Read the model definition and answer for the solid it produces. Units are mm, in the model's axes. A direction names the side the tool comes from. Round coordinates to 2 decimals unless told otherwise and drop trailing zeros. Write each loop counter-clockwise with the first axis right and the second up, starting at its lowest first coordinate (ties: lowest second). Pieces come first, ordered by that corner, then holes. Notation, with made-up numbers: M 27,16 L 42,16 A16 ccw 42,40 Z; hole C 60,87.5 d8. An arc over 180 degrees is marked long. Use one line per item in the form item = value. Start each with the question number.
```python
from build123d import *

# Parameters (mm, degrees)
SKETCH_1_R          = 1.8000000000000025
SKETCH_1_R_2        = 1.8000000000000043
SKETCH_1_R_3        = 1.8000000000000005
SKETCH_1_R_4        = 1.8000000000000007
EXTRUDE_1_DEPTH     = 42
SKETCH_2_R          = 6.000000000000001
CUT_EXTRUDE_1_DEPTH = 58.404268133998535
SKETCH_3_R          = 6.000000000000002
CUT_EXTRUDE_2_DEPTH = 58.404268133998535
SKETCH_5_W          = 12
SKETCH_5_H          = 15.000000000000005
SKETCH_5_H_2        = 15.000000000000002
CUT_EXTRUDE_3_DEPTH = 58.404268133998535
EXTRUDE_2_DEPTH     = 2.1
EXTRUDE_3_DEPTH     = 1
EXTRUDE_START       = 2.1
EXTRUDE_4_DEPTH     = 2.1
EXTRUDE_START_2     = 1
EXTRUDE_5_DEPTH     = 1
SKETCH_10_R         = 1.5000000000000018
CUT_EXTRUDE_4_DEPTH = 3


with BuildPart() as part:
    # 草图1 → 凸台-拉伸1 (new body)
    with BuildSketch(Plane(origin=(0, 0, 0), x_dir=(-1, 0, 0), z_dir=(0, 0, 1))):
        with BuildLine():
            Line((-17.499999999999996, 15), (-17.499999999999996, -15.000000000000007))
            ThreePointArc((-17.499999999999996, -15.000000000000007), (-16.767766952966365, -16.767766952966372), (-15, -17.500000000000007))
            Line((-15, -17.500000000000007), (15.000000000000004, -17.500000000000007))
            ThreePointArc((15.000000000000004, -17.500000000000007), (16.76776695296637, -16.767766952966376), (17.5, -15.00000000000001))
            Line((17.5, -15.00000000000001), (17.5, 14.999999999999996))
            ThreePointArc((17.5, 14.999999999999996), (16.76776695296637, 16.76776695296636), (15.000000000000004, 17.499999999999996))
            Line((15.000000000000004, 17.499999999999996), (-15, 17.499999999999996))
            ThreePointArc((-15, 17.499999999999996), (-16.767766952966365, 16.767766952966365), (-17.499999999999996, 15))
        make_face()
        with Locations((-15.000000000000004, -15.00000000000001)):
            Circle(SKETCH_1_R, mode=Mode.SUBTRACT)
        with Locations((15.000000000000004, -15.00000000000001)):
            Circle(SKETCH_1_R_2, mode=Mode.SUBTRACT)
        with Locations((15.000000000000004, 14.999999999999996)):
            Circle(SKETCH_1_R_3, mode=Mode.SUBTRACT)
        with Locations((-15, 15)):
            Circle(SKETCH_1_R_4, mode=Mode.SUBTRACT)
        with BuildLine():
            Line((15.604722413530899, -11.417049414734192), (15.604722413530899, 11.41704941481964))
            ThreePointArc((15.604722413530899, 11.41704941481964), (15.349600753639777, 12.084241863325458), (14.714404940145743, 12.41098197902667))
            ThreePointArc((14.714404940145743, 12.41098197902667), (13.158183898644735, 13.15818233801838), (12.410982220986185, 14.714402746377065))
            ThreePointArc((12.410982220986185, 14.714402746377065), (12.084242685294747, 15.349600017363324), (11.417049414775391, 15.604722413530212))
            Line((11.417049414775391, 15.604722413530212), (-11.417049414778536, 15.604722413530212))
            ThreePointArc((-11.417049414778536, 15.604722413530212), (-12.084241863278942, 15.349600753643644), (-12.410981978984013, 14.714404940159108))
            ThreePointArc((-12.410981978984013, 14.714404940159108), (-13.158182337972896, 13.158183898648431), (-14.714402746337697, 12.41098222098531))
            ThreePointArc((-14.714402746337697, 12.41098222098531), (-15.34960001732269, 12.084242685293246), (-15.604722413489107, 11.41704941477461))
            Line((-15.604722413489107, 11.41704941477461), (-15.604722413489107, -11.417049414779225))
            ThreePointArc((-15.604722413489107, -11.417049414779225), (-15.349600753597985, -12.084241863285039), (-14.714404940103952, -12.410981978986248))
            ThreePointArc((-14.714404940103952, -12.410981978986248), (-13.158183898602942, -13.158182337977962), (-12.410982220944396, -14.714402746336651))
            ThreePointArc((-12.410982220944396, -14.714402746336651), (-12.084242685252958, -15.34960001732291), (-11.417049414733604, -15.604722413489796))
            Line((-11.417049414733604, -15.604722413489796), (11.417049414820326, -15.604722413489796))
            ThreePointArc((11.417049414820326, -15.604722413489796), (12.084241863320731, -15.349600753603227), (12.410981979025802, -14.714404940118692))
            ThreePointArc((12.410981979025802, -14.714404940118692), (13.158182338014687, -13.158183898608014), (14.71440274637949, -12.410982220944893))
            ThreePointArc((14.71440274637949, -12.410982220944893), (15.34960001736448, -12.084242685252828), (15.604722413530899, -11.417049414734192))
        make_face(mode=Mode.SUBTRACT)
    extrude(amount=EXTRUDE_1_DEPTH)

    # 草图2 → 切除-拉伸1 (cut, through all)
    with BuildSketch(Plane(origin=(0, 17.500000000000007, 0), x_dir=(1, 0, 0), z_dir=(0, 1, 0))):
        with Locations(Location((0, -11.999999999999998, 0), (0, 0, 270))):
            Circle(SKETCH_2_R)
    extrude(amount=-CUT_EXTRUDE_1_DEPTH, mode=Mode.SUBTRACT)

    # 草图3 → 切除-拉伸2 (cut, through all)
    with BuildSketch(Plane.ZY.offset(17.5)):
        with Locations((30, 0)):
            Circle(SKETCH_3_R)
    extrude(amount=-CUT_EXTRUDE_2_DEPTH, mode=Mode.SUBTRACT)

    # 草图5 → 切除-拉伸3 (cut, through all)
    with BuildSketch(Plane(origin=(17.499999999999996, 0, 0), x_dir=(0, 0, -1), z_dir=(1, 0, 0))):
        Polygon((-30, -24.974265818952347), (-30, -15), (-42, -15), (-42, 15.000000000000007), (-30, 15.000000000000007), (-30, 23.87950348168345), (-47.41212790980853, 25.238249525472156), (-47.41212790980853, -24.974265818952347), align=None)
        with BuildLine():
            Line((-42, -15), (-30, -15))
            Line((-30, -15), (-30, -6.000000000000003))
            ThreePointArc((-29.999999999999925, -6.000000000000003), (-36, -1.93e-15), (-29.999999999999932, 6.000000000000003))
            Line((-30, 6.000000000000003), (-30, 15.000000000000007))
            Line((-30, 15.000000000000007), (-42, 15.000000000000007))
            Line((-42, 15.000000000000007), (-42, -15))
        make_face()
        with Locations((-6, 7.500000000000003)):
            Rectangle(SKETCH_5_W, SKETCH_5_H)
        Polygon((0, 15.000000000000007), (0, 0), (0, -15), (-12, -15), (-12, -24.974265818952347), (12.116605042765016, -24.974265818952347), (12.116605042765016, 23.87950348168345), (-12, 23.87950348168345), (-12, 15.000000000000007), align=None)
        with Locations((-6, -7.500000000000001)):
            Rectangle(SKETCH_5_W, SKETCH_5_H_2)
    extrude(amount=-CUT_EXTRUDE_3_DEPTH, mode=Mode.SUBTRACT)

    # 草图6 → 凸台-拉伸2 (add)
    with BuildSketch(Plane(origin=(0, 15.604722413489796, 0), x_dir=(-1, 0, 0), z_dir=(0, -1, 0))):
        with BuildLine():
            Line((-6.000000000000001, -11.999999999999998), (-6.500000000000001, -11.999999999999998))
            ThreePointArc((-6.500000000000001, -11.999999999999998), (-1.19e-15, -18.5), (6.500000000000001, -11.999999999999998))
            Line((6.500000000000001, -11.999999999999998), (6.000000000000001, -11.999999999999998))
            ThreePointArc((6.000000000000001, -11.999999999999998), (-1.1e-15, -18), (-6.000000000000001, -11.999999999999998))
        make_face()
    extrude_2 = extrude(amount=EXTRUDE_2_DEPTH)

    # 草图7 → 凸台-拉伸3 (add)
    with BuildSketch(Plane(origin=(0, 13.504722413489795, 0), x_dir=(-1, 0, 0), z_dir=(0, -1, 0))):
        with BuildLine():
            Line((-6.500000000000002, -11.999999999999998), (-5.750000000000001, -11.999999999999998))
            ThreePointArc((-5.750000000000001, -11.999999999999998), (-1.06e-15, -17.75), (5.750000000000001, -11.999999999999998))
            Line((5.750000000000001, -11.999999999999998), (6.500000000000002, -11.999999999999998))
            ThreePointArc((6.500000000000002, -11.999999999999998), (-1.19e-15, -18.5), (-6.500000000000002, -11.999999999999998))
        make_face()
    extrude_3 = extrude(amount=EXTRUDE_3_DEPTH)

    # 镜向1: 凸台-拉伸2, 凸台-拉伸3 across plane
    add(extrude_2.mirror(Plane(origin=(0, 0, 0), x_dir=(0, 0, 1), z_dir=(0, -1, 0))))
    add(extrude_3.mirror(Plane(origin=(0, 0, 0), x_dir=(0, 0, 1), z_dir=(0, -1, 0))))

    # 草图8 → 凸台-拉伸4 (add)
    with BuildSketch(Plane.ZY.offset(-15.604722413489107).offset(EXTRUDE_START)):
        with BuildLine():
            Line((30, -6.500000000000001), (30, -6.000000000000003))
            ThreePointArc((30, -6.000000000000003), (23.999999999999996, 7.3e-16), (30, 6.000000000000003))
            Line((30, 6.000000000000003), (30, 6.500000000000001))
            ThreePointArc((30, 6.500000000000001), (23.5, 8e-16), (30, -6.500000000000001))
        make_face()
    extrude_4 = extrude(amount=-EXTRUDE_4_DEPTH)

    # 草图9 → 凸台-拉伸5 (add)
    with BuildSketch(Plane.ZY.offset(-13.504722413489107).offset(EXTRUDE_START_2)):
        with BuildLine():
            Line((30, -6.500000000000001), (30, -5.750000000000003))
            ThreePointArc((30, -5.750000000000003), (24.249999999999996, 7e-16), (30, 5.750000000000003))
            Line((30, 5.750000000000003), (30, 6.500000000000001))
            ThreePointArc((30, 6.500000000000001), (23.5, 8e-16), (30, -6.500000000000001))
        make_face()
    extrude_5 = extrude(amount=-EXTRUDE_5_DEPTH)

    # 镜向2: 凸台-拉伸4, 凸台-拉伸5 across plane
    add(extrude_4.mirror(Plane.ZY))
    add(extrude_5.mirror(Plane.ZY))

    # 草图10 → 切除-拉伸4 (cut)
    with BuildSketch(Plane.XZ.offset(17.499999999999996)):
        with Locations(Location((-1.8416814e-09, 23.000000000000025, 0), (0, 0, 270))):
            Circle(SKETCH_10_R)
    extrude(amount=-CUT_EXTRUDE_4_DEPTH, mode=Mode.SUBTRACT)


solid = part.part
```
Q1. Find section D-D on x = -8. Write down the section's boundary in (y, z).
Q2. Straight lines are drawn through the part: line 1 (X direction, y = 4, z = 13.5); line 2 (Y direction, x = -15, z = 17.5). For each, find the intervals that lie inside material, in ascending order. Write a range as [from, to].
Q3. Find section B-B on z = 23. Count the separate pieces of the cut face and the enclosed holes in it, and give its area (3 significant figures).
Q4. For a pull along Y with two mould halves and no side action, classify faces 4 (the face through (0, -17.5, 21)), 5 (the face through (-13, -0.13, 24.25)), 6 (the face through (0.13, 13.01, 17.75)) as +Y half, -Y half, draft (parallel to the pull), parting line (faces both ways), or undercut.
Q5. Find section A-A on x = 0. Write down the section's boundary in (y, z), and give its area (3 significant figures).
Q6. A tool of negligible diameter and unlimited length cuts with its end or side. For faces 1 (the face through (12.505, 0, 24)), 2 (the face through (15.605, 0, 19)), 3 (the face through (16.748, -16.787, 20.874)), from which of +Z, -Z, +X, -X, +Y, -Y can it reach the whole face along a straight path? Write none if from no direction.
Q7. Find section C-C on y = 0. Write down the section's boundary in (x, z), and give its area (3 significant figures).
Q8. This flat-tipped pin is pushed along its axis until it touches: pin 1 Ø6.5 at (y, z) = (1, 27.5) entering from -X. Where does it stop, or does it pass through?
Response:
q1.outline = M -17.5,12 L -15.6,12 L -15.6,30 L -17.5,30 Z; M 15.6,12 L 17.5,12 L 17.5,30 L 15.6,30 Z
q2.line_1 = [-17.5, -15.6], [15.6, 17.5]
q2.line_2 = [-17.5, -16.8], [-13.2, -12.34], [12.34, 13.2], [16.8, 17.5]
q3.separate_pieces = 1
q3.enclosed_holes = 4
q3.area = 236 mm²
q4.face_4 = -Y half
q4.face_5 = undercut
q4.face_6 = draft
q5.outline = M -17.5,18 L -13.5,18 L -13.5,17.75 L -12.5,17.75 L -12.5,18.5 L -15.6,18.5 L -15.6,21.5 L -17.5,21.5 Z; M -17.5,24.5 L -15.6,24.5 L -15.6,30 L -17.5,30 Z; M 12.5,17.75 L 13.5,17.75 L 13.5,18 L 17.5,18 L 17.5,30 L 15.6,30 L 15.6,18.5 L 12.5,18.5 Z
q5.area = 43.4 mm²
q6.face_1 = +Z, -Z
q6.face_2 = -Z
q6.face_3 = +Z, -Z, +X, -Y
q7.outline = M -17.5,12 L -15.6,12 L -15.6,23.5 L -12.5,23.5 L -12.5,24.25 L -13.5,24.25 L -13.5,24 L -17.5,24 Z; M 12.5,23.5 L 15.6,23.5 L 15.6,12 L 17.5,12 L 17.5,24 L 13.5,24 L 13.5,24.25 L 12.5,24.25 Z
q7.area = 49.1 mm²
q8.pin_1 = -13.5
